```python
from build123d import *

# Parameters (mm, degrees)
F0_W     = 15
F0_H     = 15
F1_DEPTH = 15
F2_W     = 5
F2_H     = 5
F3_DEPTH = 10
F2_R     = 1.5
F4_DEPTH = 5
F2_W_2   = 3
F2_H_2   = 3
F5_DEPTH = 10
F6_SIZE  = 5
F8_DEPTH = 5
F9_SIZE  = 1


with BuildPart() as f1:
    # F0 (on Top) → F1 (new body)
    with BuildSketch(Plane.XY):
        with Locations((7.5, 0)):
            Rectangle(F0_W, F0_H)
    extrude(amount=F1_DEPTH)

    # F2 (on face) → F3 (join)
    with BuildSketch(Plane.XY.offset(15)):
        with Locations((2.5, -5)):
            Rectangle(F2_W, F2_H)
    extrude(amount=F3_DEPTH)

    # F2 (on face) → F4 (join)
    with BuildSketch(Plane.XY.offset(15)):
        with Locations((10, -3)):
            Circle(F2_R)
    extrude(amount=F4_DEPTH)

    # F2 (on face) → F5 (cut)
    with BuildSketch(Plane.XY.offset(15)):
        with Locations((13.5, 6)):
            Rectangle(F2_W_2, F2_H_2)
    extrude(amount=-F5_DEPTH, mode=Mode.SUBTRACT)

    # F6
    f6_edges = [f1.edges().sort_by_distance(p)[0] for p in [
        (0, 2.5, 15),
    ]]
    chamfer(f6_edges, length=F6_SIZE)

    # F7 (on face) → F8 (join)
    with BuildSketch(Plane.XZ.offset(7.5)):
        Polygon((24.155803, 15), (15, 15), (15, 5.844197), align=None)
    extrude(amount=-F8_DEPTH)

    # F9
    f9_edges = [f1.edges().sort_by_distance(p)[0] for p in [
        (8.5, -3, 20),
    ]]
    chamfer(f9_edges, length=F9_SIZE)


solid = f1.part
```
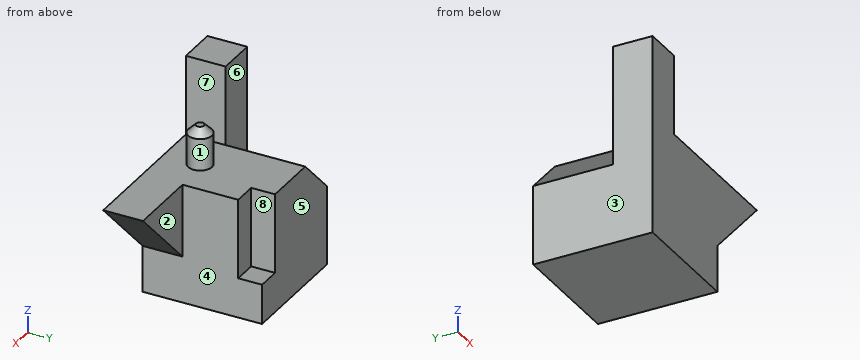
Geometry: final body of the model. Coordinates: model frame, mm. Face numbers are marked on the shaded views. A direction names the side the tool comes from. Coordinates: 2 decimals unless noted, no trailing zeros. Order: outer loops, then holes, each group sorted by start corner. A loop starts at its lowest first (then second) coordinate and runs counter-clockwise, first axis right, second up.
Item 1: Draft query along X for the marked faces 1, 2 and 3. Return one class per face: released by +X, released by -X, zero draft, split by the parting line, or undercut.
Answer:
face 1: undercut
face 2: zero draft
face 3: released by -X
Item 2: Contact query for flat-ended pins moving along their axis: P1, Ø4, axis at x = 2.5, z = 16.5, coming from the +Y side; P2, Ø2.5, axis at x = 14, y = 6.5, coming from the +Z side; P3, Ø1.5, axis at y = 5.5, z = 10.5, coming from the +X side; P4, Ø3, axis at x = 2.5, y = -3, coming from the -Z side. Output: stop coordinate, or through.
Answer:
P1: stops at y = -2.5
P2: stops at z = 5
P3: stops at x = 12
P4: stops at z = 0
Item 3: Section query D-D (x = 3.5). Output: boundary loops of the cut face in (y, z).
Answer:
outline: (-7.5, 0) - (7.5, 0) - (7.5, 13.5) - (-2.5, 13.5) - (-2.5, 25) - (-7.5, 25) - close
Item 4: Section query C-C (z = 8.25). Output: boundary loops of the cut face in (x, y), then the cut area to 3 significant figures.
Answer:
outline: (0, -7.5) - (17.41, -7.5) - (17.41, -2.5) - (15, -2.5) - (15, 4.5) - (12, 4.5) - (12, 7.5) - (0, 7.5) - close
area: 228 mm2
Item 5: Material intervals for line 1 along X through (y, z) = (-2, 14.5); line 2 along X through (y, z) = (-3, 20.5); line 3 along Z through (x, y) = (5.5, 1.5), sorted ascending.
Answer:
line 1: x = 4.5 to 15
line 2: x = 0 to 5
line 3: z = 0 to 15
Item 6: Section query A-A (x = 10). Output: boundary loops of the cut face in (y, z), then the cut area to 3 significant figures.
Answer:
outline: (-7.5, 0) - (7.5, 0) - (7.5, 15) - (-1.5, 15) - (-1.5, 19) - (-2.5, 20) - (-3.5, 20) - (-4.5, 19) - (-4.5, 15) - (-7.5, 15) - close
area: 239 mm2
Item 7: Section query B-B (y = -5). Output: boundary loops of the cut face in (x, z), then the cut area to 3 significant figures.
Answer:
outline: (0, 0) - (15, 0) - (15, 5.84) - (24.16, 15) - (5, 15) - (5, 25) - (0, 25) - close
area: 317 mm2
Item 8: Access query for the marked faces 4, 5, 6, 7 and 8. Directions: +Z, -Z, +X, -X, +Y, -Y. A direction counts if a zero-diameter tool reaches every point of the face in a straight line with its end or side. Return the directions, or none.
Answer:
face 4: -Z, +X, +Y
face 5: +Z, -Z, +X, -X, +Y
face 6: +Z, -X, +Y
face 7: +Z, +Y, -Y
face 8: +Z, +X, +Y
